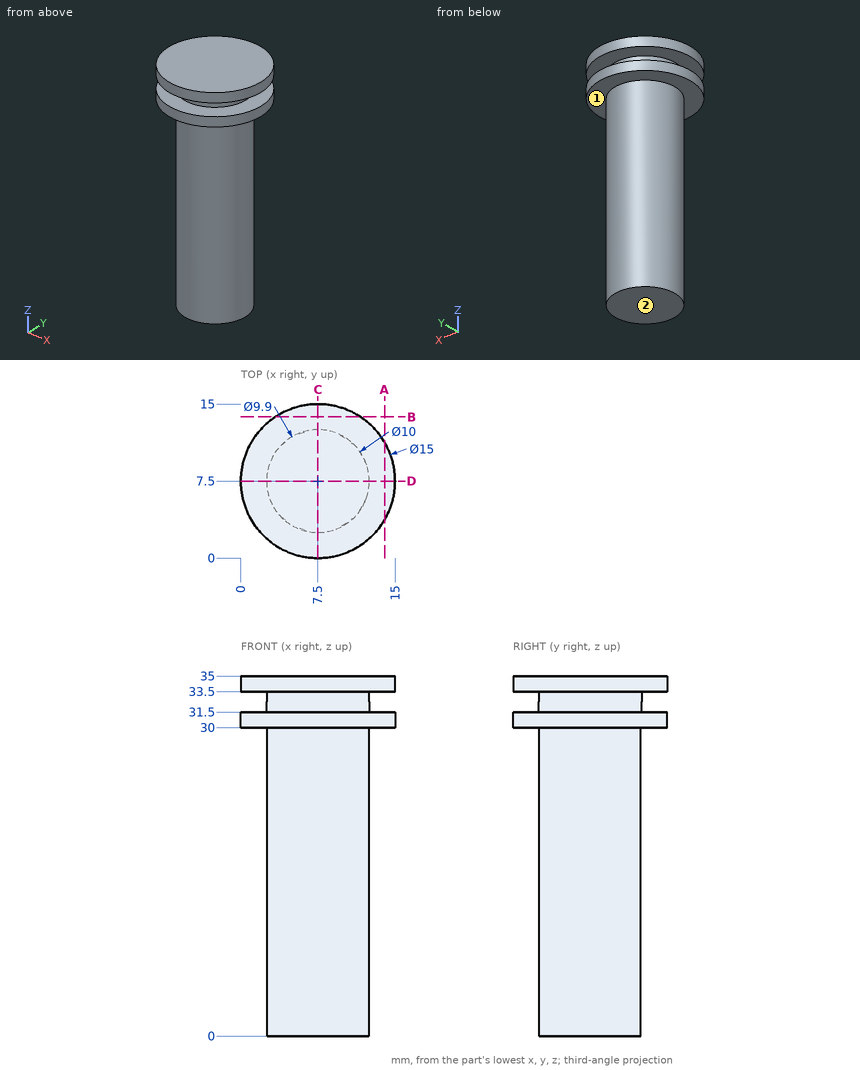
Print and shaded views of the part. All mm, measured from the part's lowest x, y and z. A direction names the side the tool comes from. Round coordinates to 2 decimals unless told otherwise and drop trailing zeros. Write each loop counter-clockwise with the first axis right and the second up, starting at its lowest first coordinate (ties: lowest second). Pieces come first, ordered by that corner, then holes. Notation, with made-up numbers: M -9,24 L 40,24 A12 ccw 40,28 Z; hole C 29.5,41 d8. An arc over 180 degrees is marked long. Use a Markdown table: item, result. Add a question column.
1. Drill centre lines: probe 1 along Z at (x, y) = (13.5, 11.25); probe 2 along X at (y, z) = (7.5, 21); probe 3 along Y at (x, z) = (3.25, 15.5). Where is each one in solid material? Low to high.
2. Flat gauge pins, fed straight in: P1, Ø5, axis at x = 7.5, z = 19, coming from the +Y side; P2, Ø6, axis at y = 11, z = 26.5, coming from the -X side; P3, Ø4, axis at x = 10.5, z = 24.5, coming from the +Y side. Where does each tip first touch, or does it go through?
3. Slice it at A-A on x = 14. Give the cut face in (y, z).
4. 3-axis set-ups, long thin cutter, end or side, ignore diameter. For the marked faces 1 and 2: which of +Z, -Z, +X, -X, +Y, -Y reach the whole face in a straight line?
5. Slice it at B-B on y = 13.75. Give the cut face in (x, z).
6. Slice it at C-C on x = 7.5. Give the cut face in (y, z), then the cut area to 3 significant figures.
Reply:
| question | item | result |
|---|---|---|
| 1 | probe 1 | z = 30 to 31.5, 33.5 to 35 |
| 1 | probe 2 | x = 2.55 to 12.45 |
| 1 | probe 3 | y = 4.96 to 10.04 |
| 2 | P1 | stops at y = 12.45 |
| 2 | P2 | stops at x = 2.58 |
| 2 | P3 | stops at y = 12.35 |
| 3 | outline | M 3.76,30 L 11.24,30 L 11.24,31.5 L 3.76,31.5 Z; M 3.76,33.5 L 11.24,33.5 L 11.24,35 L 3.76,35 Z |
| 4 | face 1 | -Z |
| 4 | face 2 | -Z, +X, -X, +Y, -Y |
| 5 | outline | M 3.35,30 L 11.65,30 L 11.65,31.5 L 3.35,31.5 Z; M 3.35,33.5 L 11.65,33.5 L 11.65,35 L 3.35,35 Z |
| 6 | outline | M 0,30 L 2.55,30 L 2.55,0 L 12.45,0 L 12.45,30 L 15,30 L 15,31.5 L 12.5,31.5 L 12.5,33.5 L 15,33.5 L 15,35 L 0,35 L 0,33.5 L 2.5,33.5 L 2.5,31.5 L 0,31.5 Z |
| 6 | area | 362 mm^2 |
